Job drawing, mm, ordinate dimensions from the low corner. One solid piece. A direction names the side the tool comes from. Round coordinates to 2 decimals unless told otherwise and drop trailing zeros. Order: outer loops, then holes, each group sorted by start corner. A loop starts at its lowest first (then second) coordinate and runs counter-clockwise, first axis right, second up. Notation, with made-up numbers: (55, 45.5) -> (75, 45.5) arc R23 cw to (75, 69.5) -> close; hole circle Ø7 at (-11.5, -12). An arc over 180 degrees is marked (long way). Write item = value, one per line.
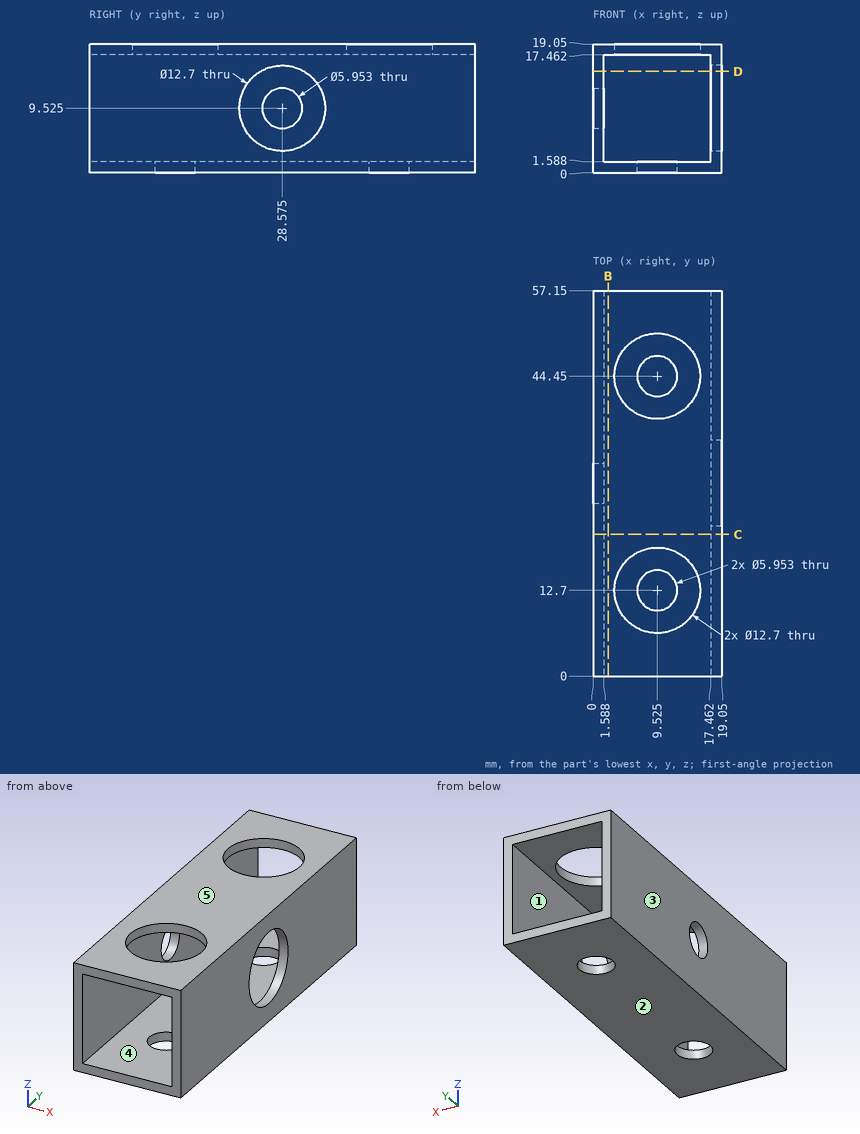
Q1. Which spindle directions (+Z, -Z, +X, -X, +Y, -Y) get a long thin tool onto all of the face, cutting with end or side? Do the marked faces 4 and 5. Say none if no direction does.
Check values:
face_4 = +Y, -Y
face_5 = +Z, +X, -X, +Y, -Y
Q2. Cut at D-D, the plane z = 15. List the corners of the cut face in (x, y).
Check values:
outline = (0, 0) -> (1.59, 0) -> (1.59, 57.15) -> (0, 57.15) -> close; (17.46, 0) -> (19.05, 0) -> (19.05, 25.36) -> (17.46, 25.36) -> close; (17.46, 31.79) -> (19.05, 31.79) -> (19.05, 57.15) -> (17.46, 57.15) -> close
Q3. Probe probe 1 along X at (y, z) = (38.5, 12.75); probe 2 along X at (y, z) = (44.45, 0.95). List the from-to ranges inside material, lowest first.
Check values:
probe_1 = 0 to 1.59, 17.46 to 19.05
probe_2 = 0 to 6.55, 12.5 to 19.05
Q4. Cut at C-C, the plane y = 21. List the corners of the cut face in (x, z), and give its area (3 significant figures).
Check values:
outline = (0, 0) -> (19.05, 0) -> (19.05, 19.05) -> (0, 19.05) -> close; hole (1.59, 1.59) -> (17.46, 1.59) -> (17.46, 17.46) -> (1.59, 17.46) -> close
area = 111 mm²
Q5. Flat gauge pins, fed straight in: pin 1 (9.5 mm diameter, centred on x = 9.525, y = 44.45, fed in from +Z); pin 2 (6 mm diameter, centred on x = 3.5, z = 5, fed in from +Y); pin 3 (9.5 mm diameter, centred on y = 28.575, z = 9.525, fed in from +X). Where does each tip first touch, or does it go through?
Check values:
pin_1 = 1.59
pin_2 = 57.15
pin_3 = 1.59
Q6. Mould opens along X. For the marked faces 1, 2 and 3 say: released by +X, released by -X, zero draft, split by the parting line, or undercut.
Check values:
face_1 = undercut
face_2 = zero draft
face_3 = released by -X
Q7. Cut at B-B, the plane x = 2.25. List the corners of the cut face in (y, z).
Check values:
outline = (0, 0) -> (57.15, 0) -> (57.15, 1.59) -> (0, 1.59) -> close; (0, 17.46) -> (57.15, 17.46) -> (57.15, 19.05) -> (0, 19.05) -> close
